Answer from the drawing. Dimensions are ordinates in mm from the lowest x, y and z of the part. A direction names the side the tool comes from. Give positions to 0.01 mm unless a question says otherwise; leave off trailing zeros. Loops run counter-clockwise (first coordinate to the right, second up) from the corner with the lowest first, then second, coordinate; pieces in that order, holes last.
(1) Find section D-D, the plane y = 9. Write down the section's boundary in (x, z).
(2) Which of the six approach directions +Z, -Z, +X, -X, +Y, -Y give full straight-line access (tool end or side, diameter ignored) to the marked faces 1 and 2?
(3) Determine the mould class of the marked faces 3, 4 and 5 for opening direction Y: pulls with the +Y half, pulls with the -Y half, needs draft (parallel to the pull), parting line crosses it, or undercut.
(4) Find section B-B, the plane z = 41.5. Write down the section's boundary in (x, y), then the cut area to 3 significant figures.
(5) Find section C-C, the plane z = 8. Write down the section's boundary in (x, y), then the cut area to 3 significant figures.
(6) Each of these flat-tipped pins is pushed along its axis until it touches: P1, Ø4, axis at x = 43, y = 11, coming from the +Z side; P2, Ø11.5, axis at x = 38.5, y = 28.5, coming from the -Z side; P3, Ø10, axis at x = 44, z = 14.5, coming from the -Y side. Where does it stop, or does it pass through?
(7) Find section A-A, the plane x = 16. Write down the section's boundary in (y, z), then the cut area to 3 significant figures.
(8) Straight lines are drawn through the part: probe 1 along Y at (x, z) = (53, 37.5); probe 2 along Y at (x, z) = (15, 15); probe 3 along Z at (x, y) = (7, 15). For each, find the intervals that lie inside material, in ascending order.
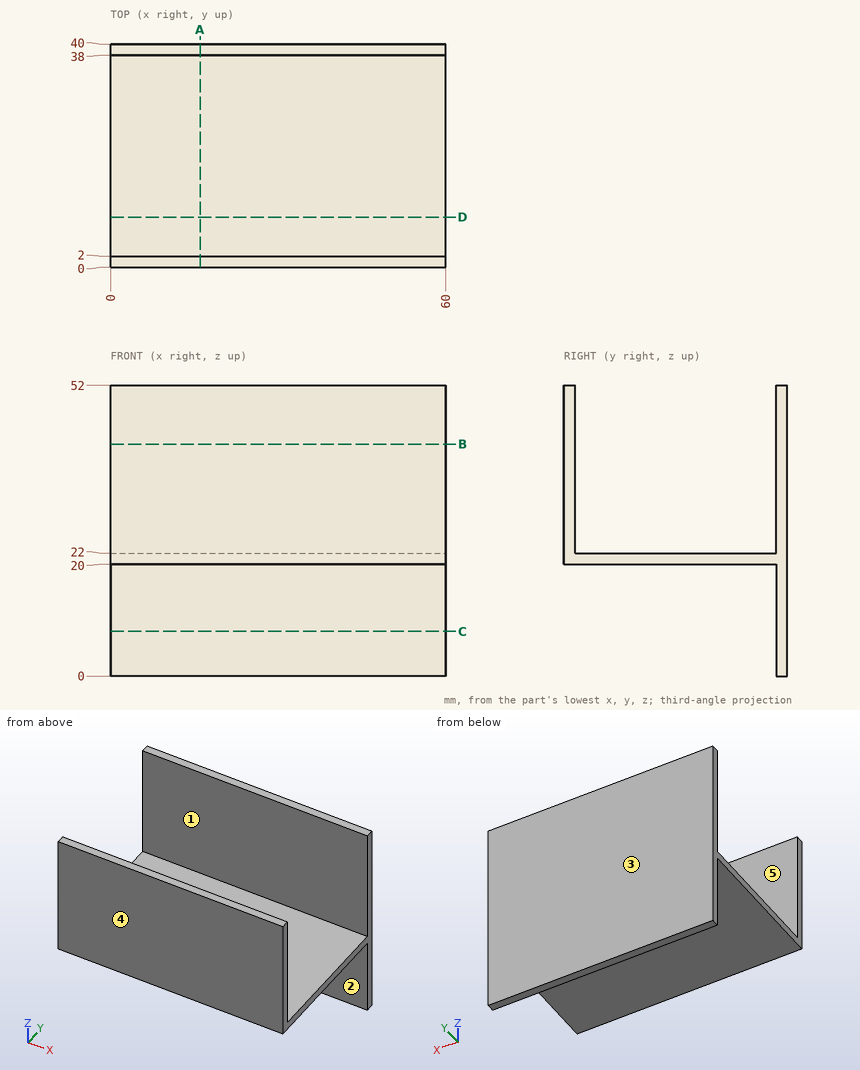
Entries:
1. outline: (0, 20) - (60, 20) - (60, 22) - (0, 22) - close
2. face 1: +Z, +X, -X
2. face 2: -Z, +X, -X, -Y
3. face 3: pulls with the +Y half
3. face 4: pulls with the -Y half
3. face 5: undercut
4. outline: (0, 0) - (60, 0) - (60, 2) - (0, 2) - close; (0, 38) - (60, 38) - (60, 40) - (0, 40) - close
4. area: 240 mm2
5. outline: (0, 38) - (60, 38) - (60, 40) - (0, 40) - close
5. area: 120 mm2
6. P1: stops at z = 22
6. P2: stops at z = 20
6. P3: stops at y = 38
7. outline: (0, 20) - (38, 20) - (38, 0) - (40, 0) - (40, 52) - (38, 52) - (38, 22) - (2, 22) - (2, 52) - (0, 52) - close
7. area: 240 mm2
8. probe 1: y = 0 to 2, 38 to 40
8. probe 2: y = 38 to 40
8. probe 3: z = 20 to 22
